Geometry check sheet. Reference: the model listing, model coordinates, mm. Round coordinates to 2 decimals unless told otherwise and drop trailing zeros. Write each loop counter-clockwise with the first axis right and the second up, starting at its lowest first coordinate (ties: lowest second). Pieces come first, ordered by that corner, then holes. Notation, with made-up numbers: (75, 21) - (118, 21) arc R22 ccw to (118, 50) - close; hole circle Ø3 at (70, 20). An arc over 180 degrees is marked (long way). Return JSON: item names as keys, results as strings.
```python
from build123d import *

# Parameters (mm, degrees)
F0_W     = 50.8
F0_H     = 69.85
F1_DEPTH = 25.4
F2_R     = 9.525
F3_DEPTH = 25.401
F4_SIZE  = 9.525
F5_SIZE  = 0.79375


with BuildPart() as f1:
    # F0 (on Right) → F1 (new body)
    with BuildSketch(Plane.YZ):
        with Locations((25.4, 34.925)):
            Rectangle(F0_W, F0_H)
    extrude(amount=F1_DEPTH)

    # F2 (on face) → F3 (cut, through all)
    with BuildSketch(Plane.YZ.offset(25.4)):
        with Locations((25.4, 47.625)):
            Circle(F2_R)
    extrude(amount=-F3_DEPTH, mode=Mode.SUBTRACT)

    # F4
    f4_edges = [f1.edges().sort_by_distance(p)[0] for p in [
        (12.7, 50.8, 69.85),
        (12.7, 0, 69.85),
    ]]
    chamfer(f4_edges, length=F4_SIZE)

    # F5
    f5_edges = [f1.edges().sort_by_distance(p)[0] for p in [
        (0, 15.875, 47.625),
        (25.4, 15.875, 47.625),
    ]]
    chamfer(f5_edges, length=F5_SIZE)


solid = f1.part
```
(1) Section check C-C, the plane y = 46.5. Enter the section's corners in (x, z) (3 decimals), plus the area to 3 significant figures.
Response values:
{"outline": "(0, 0) - (25.4, 0) - (25.4, 64.625) - (0, 64.625) - close", "area": "1,640 mm^2"}
(2) Section check B-B, the plane x = 12.75. Enter the section's corners in (y, z) (3 decimals), plus the area to 3 significant figures.
Response values:
{"outline": "(0, 0) - (50.8, 0) - (50.8, 60.325) - (41.275, 69.85) - (9.525, 69.85) - (0, 60.325) - close; hole circle Ø19.05 at (25.4, 47.625)", "area": "3,170 mm^2"}
(3) Release check for a two-part mould opening along Y. For faces 1 (the face through (12.867, 23.335, 38.327)), 2 (the face through (13, 25, 69.85)), 3 (the face through (12.522, 46.104, 65.021)) record: pulls with the +Y half, pulls with the -Y half, needs draft (parallel to the pull), parting line crosses it, or undercut.
Response values:
{"face 1": "undercut", "face 2": "needs draft", "face 3": "pulls with the +Y half"}
(4) Material ranges on line 1 along Z through (x, y) = (19.25, 25.4); line 2 along Y through (x, z) = (19, 46); line 3 along Z through (x, y) = (2, 31.5), recorded low to high. Write a range as [from, to].
Response values:
{"line 1": "z = [0, 38.1], [57.15, 69.85]", "line 2": "y = [0, 16.01], [34.79, 50.8]", "line 3": "z = [0, 40.31], [54.94, 69.85]"}
(5) Section check A-A, the plane y = 25.4. Enter the section's corners in (x, z), plus the area to 3 significant figures.
Response values:
{"outline": "(0, 0) - (25.4, 0) - (25.4, 37.31) - (24.61, 38.1) - (0.79, 38.1) - (0, 37.31) - close; (0, 57.94) - (0.79, 57.15) - (24.61, 57.15) - (25.4, 57.94) - (25.4, 69.85) - (0, 69.85) - close", "area": "1,290 mm^2"}
